Part model, mm, in its own coordinate system. A direction names the side the tool comes from. Give positions to 0.01 mm unless a question says otherwise; leave off trailing zeros. Order: outer loops, then holes, each group sorted by start corner. A loop starts at its lowest first (then second) coordinate and runs counter-clockwise, first axis right, second up. Notation, with made-up numbers: (-6, 71) - (27, 71) arc R15 ccw to (27, 97) - close; hole circle Ø3 at (-27.75, 81.5). An arc over 180 degrees is marked (long way). Use one line per item in the form item = value. Start each with the question number.
1. Pin check, flat tips, straight feed: P1, Ø1.5, axis at x = 13.5, z = 2, coming from the +Y side; P2, Ø1, axis at x = -8.5, z = 2.5, coming from the +Y side; P3, Ø1.5, axis at x = 33.5, z = 3, coming from the +Y side. Stop position of each tip, or through.
2. Tool access for faces 3 (the face through (59, 39, 1)), 4 (the face through (14, 43, 4)): list every direction of +Z, -Z, +X, -X, +Y, -Y with a clear straight run to the whole face (end or side of a thin tool).
3. Pull direction X, two halves, no side cores. Call faces 1 (the face through (-17.24, 37.82, 2.48)), 2 (the face through (14, 43, 0)): +X half, -X half, draft (parallel to the pull), parting line (faces both ways), or undercut.
4. Band-saw the part on B-B, the plane y = 25.5. List the corners of the cut face in (x, z), plus the area to 3 significant figures.
5. Drill centre lines: line 1 (X direction, y = 31.5, z = 1.15); line 2 (Y direction, x = 48, z = 3.4); line 3 (X direction, y = 30, z = 2.5). Where is each one in solid material? Low to high.
6. Band-saw the part on A-A, the plane z = 2. List the corners of the cut face in (x, y), plus the area to 3 significant figures.
from build123d import *

# Parameters (mm, degrees)
F1_DEPTH = 4
F2_DEPTH = 1


with BuildPart() as f1:
    # F0 (on Top) → F1 (new body)
    with BuildSketch(Plane.XY):
        with BuildLine():
            ThreePointArc((33.96875, 44.7240123715), (35.4798914594, 41.6976549267), (36, 38.3552194374))
            ThreePointArc((36, 38.3552194374), (35.4798914594, 35.0127839481), (33.96875, 31.9864265033))
            ThreePointArc((33.96875, 31.9864265033), (34.890304672, 30.0329837344), (36.04875, 28.2100174464))
            ThreePointArc((36.04875, 28.2100174464), (38.9773253879, 32.9114730252), (40, 38.3552194374))
            ThreePointArc((40, 38.3552194374), (38.9773253879, 43.7989658495), (36.04875, 48.5004214283))
            ThreePointArc((36.04875, 48.5004214283), (34.890304672, 46.6774551404), (33.96875, 44.7240123715))
        make_face()
        with BuildLine():
            ThreePointArc((31.92, 46.9058685355), (33.0189287452, 45.8849459782), (33.96875, 44.7240123715))
            ThreePointArc((33.96875, 44.7240123715), (34.890304672, 46.6774551404), (36.04875, 48.5004214283))
            ThreePointArc((36.04875, 48.5004214283), (35.0671824784, 49.4751041915), (34, 50.3552194374))
            ThreePointArc((34, 50.3552194374), (32.8729423014, 48.6830408238), (31.92, 46.9058685355))
        make_face()
        with BuildLine():
            ThreePointArc((36.04875, 28.2100174464), (34.890304672, 30.0329837344), (33.96875, 31.9864265033))
            ThreePointArc((33.96875, 31.9864265033), (33.0189287452, 30.8254928966), (31.92, 29.8045703392))
            ThreePointArc((31.92, 29.8045703392), (32.8729423014, 28.027398051), (34, 26.3552194374))
            ThreePointArc((34, 26.3552194374), (35.0671824784, 27.2353346832), (36.04875, 28.2100174464))
        make_face()
        with BuildLine():
            ThreePointArc((18.08, 46.9058685355), (25, 49.3552194374), (31.92, 46.9058685355))
            ThreePointArc((31.92, 46.9058685355), (32.8729423014, 48.6830408238), (34, 50.3552194374))
            ThreePointArc((34, 50.3552194374), (25, 53.3552194374), (16, 50.3552194374))
            ThreePointArc((16, 50.3552194374), (17.1270576986, 48.6830408238), (18.08, 46.9058685355))
        make_face()
        with BuildLine():
            ThreePointArc((39.8607042186, 52.31076246), (37.804989803, 50.5553926449), (36.04875, 48.5004214283))
            ThreePointArc((36.04875, 48.5004214283), (38.9773253879, 43.7989658495), (40, 38.3552194374))
            ThreePointArc((40, 38.3552194374), (38.9773253879, 32.9114730252), (36.04875, 28.2100174464))
            ThreePointArc((36.04875, 28.2100174464), (37.8049899077, 26.1550461251), (39.8607044582, 24.3996762406))
            ThreePointArc((39.8607044582, 24.3996762406), (38.8098535793, 31.0344868958), (45.4446642345, 32.0853377748))
            ThreePointArc((45.4446642345, 32.0853377748), (42.25, 38.3552195837), (45.4446644712, 44.625101272))
            ThreePointArc((45.4446644712, 44.625101272), (38.8098537523, 45.6759517408), (39.8607042186, 52.31076246))
        make_face()
        with BuildLine():
            ThreePointArc((34, 50.3552194374), (35.0671824784, 49.4751041915), (36.04875, 48.5004214283))
            ThreePointArc((36.04875, 48.5004214283), (37.804989803, 50.5553926449), (39.8607042186, 52.31076246))
            ThreePointArc((39.8607042186, 52.31076246), (57.8313360218, 53.7250820299), (67.25, 38.3552194374))
            ThreePointArc((67.25, 38.3552194374), (57.8313361537, 22.985356912), (39.8607044582, 24.3996762406))
            ThreePointArc((39.8607044582, 24.3996762406), (37.8049899077, 26.1550461251), (36.04875, 28.2100174464))
            ThreePointArc((36.04875, 28.2100174464), (35.0671824784, 27.2353346832), (34, 26.3552194374))
            ThreePointArc((34, 26.3552194374), (37.3874296651, 22.8335227019), (41.5277360562, 20.2383559211))
            ThreePointArc((41.5277360562, 20.2383559211), (43.9514682435, 19.5144497823), (46.3436548255, 18.6922812041))
            ThreePointArc((46.3436548255, 18.6922812041), (62.7842304522, 22.9746000823), (70, 38.3552194374))
            ThreePointArc((70, 38.3552194374), (62.7842304522, 53.7358387924), (46.3436548255, 58.0181576706))
            ThreePointArc((46.3436548255, 58.0181576706), (43.9514682435, 57.1959890924), (41.5277360562, 56.4720829536))
            ThreePointArc((41.5277360562, 56.4720829536), (37.3874296651, 53.8769161728), (34, 50.3552194374))
        make_face()
        with BuildLine():
            ThreePointArc((34, 26.3552194374), (32.8729423014, 28.027398051), (31.92, 29.8045703392))
            ThreePointArc((31.92, 29.8045703392), (25, 27.3552194374), (18.08, 29.8045703392))
            ThreePointArc((18.08, 29.8045703392), (17.1270576986, 28.027398051), (16, 26.3552194374))
            ThreePointArc((16, 26.3552194374), (25, 23.3552194374), (34, 26.3552194374))
        make_face()
        with BuildLine():
            ThreePointArc((16.03125, 44.7240123715), (16.9810712548, 45.8849459782), (18.08, 46.9058685355))
            ThreePointArc((18.08, 46.9058685355), (17.1270576986, 48.6830408238), (16, 50.3552194374))
            ThreePointArc((16, 50.3552194374), (14.9328175216, 49.4751041915), (13.95125, 48.5004214283))
            ThreePointArc((13.95125, 48.5004214283), (15.109695328, 46.6774551404), (16.03125, 44.7240123715))
        make_face()
        with BuildLine():
            ThreePointArc((16, 50.3552194374), (25, 53.3552194374), (34, 50.3552194374))
            ThreePointArc((34, 50.3552194374), (37.3874296651, 53.8769161728), (41.5277360562, 56.4720829536))
            ThreePointArc((41.5277360562, 56.4720829536), (25, 54.228538177), (8.4722639438, 56.4720829536))
            ThreePointArc((8.4722639438, 56.4720829536), (12.6125703349, 53.8769161728), (16, 50.3552194374))
        make_face()
        with BuildLine():
            ThreePointArc((16, 26.3552194374), (17.1270576986, 28.027398051), (18.08, 29.8045703392))
            ThreePointArc((18.08, 29.8045703392), (16.9810712548, 30.8254928966), (16.03125, 31.9864265033))
            ThreePointArc((16.03125, 31.9864265033), (15.109695328, 30.0329837344), (13.95125, 28.2100174464))
            ThreePointArc((13.95125, 28.2100174464), (14.9328175216, 27.2353346832), (16, 26.3552194374))
        make_face()
        with BuildLine():
            ThreePointArc((41.5277360562, 20.2383559211), (37.3874296651, 22.8335227019), (34, 26.3552194374))
            ThreePointArc((34, 26.3552194374), (25, 23.3552194374), (16, 26.3552194374))
            ThreePointArc((16, 26.3552194374), (12.6125703349, 22.8335227019), (8.4722639438, 20.2383559211))
            ThreePointArc((8.4722639438, 20.2383559211), (25, 22.4819006978), (41.5277360562, 20.2383559211))
        make_face()
        with BuildLine():
            ThreePointArc((16.03125, 31.9864265033), (14, 38.3552194374), (16.03125, 44.7240123715))
            ThreePointArc((16.03125, 44.7240123715), (15.109695328, 46.6774551404), (13.95125, 48.5004214283))
            ThreePointArc((13.95125, 48.5004214283), (10, 38.3552194374), (13.95125, 28.2100174464))
            ThreePointArc((13.95125, 28.2100174464), (15.109695328, 30.0329837344), (16.03125, 31.9864265033))
        make_face()
        with BuildLine():
            ThreePointArc((13.95125, 48.5004214283), (14.9328175216, 49.4751041915), (16, 50.3552194374))
            ThreePointArc((16, 50.3552194374), (12.6125703349, 53.8769161728), (8.4722639438, 56.4720829536))
            ThreePointArc((8.4722639438, 56.4720829536), (6.0485317565, 57.1959890924), (3.6563451745, 58.0181576706))
            ThreePointArc((3.6563451745, 58.0181576706), (-20, 38.3552194374), (3.6563451745, 18.6922812041))
            ThreePointArc((3.6563451745, 18.6922812041), (6.0485317565, 19.5144497823), (8.4722639438, 20.2383559211))
            ThreePointArc((8.4722639438, 20.2383559211), (12.6125703349, 22.8335227019), (16, 26.3552194374))
            ThreePointArc((16, 26.3552194374), (14.9328175216, 27.2353346832), (13.95125, 28.2100174464))
            ThreePointArc((13.95125, 28.2100174464), (12.1950101323, 26.1550461651), (10.1392956333, 24.3996763071))
            ThreePointArc((10.1392956333, 24.3996763071), (-17.25, 38.3552194393), (10.1392956365, 52.3107625653))
            ThreePointArc((10.1392956365, 52.3107625653), (12.1950101337, 50.5553927082), (13.95125, 48.5004214283))
        make_face()
        with BuildLine():
            ThreePointArc((50, 46.1052194374), (47.6051183973, 45.7259074724), (45.4446644712, 44.625101272))
            ThreePointArc((45.4446644712, 44.625101272), (42.25, 38.3552195837), (45.4446642345, 32.0853377748))
            ThreePointArc((45.4446642345, 32.0853377748), (53.5184263398, 31.449918858), (57.75, 38.3552194374))
            ThreePointArc((57.75, 38.3552194374), (55.4800775542, 43.8352969916), (50, 46.1052194374))
        make_face()
        with BuildLine():
            ThreePointArc((13.95125, 28.2100174464), (10, 38.3552194374), (13.95125, 48.5004214283))
            ThreePointArc((13.95125, 48.5004214283), (12.1950101337, 50.5553927082), (10.1392956365, 52.3107625653))
            ThreePointArc((10.1392956365, 52.3107625653), (11.5795966532, 50.6243867219), (12.0973156537, 48.4679318671))
            ThreePointArc((12.0973156537, 48.4679318671), (9.503770504, 44.2356508652), (4.5553356627, 44.6251011747))
            ThreePointArc((4.5553356627, 44.6251011747), (6.9053005505, 41.8736458338), (7.75, 38.3552194374))
            ThreePointArc((7.75, 38.3552194374), (6.9053005928, 34.8367931239), (4.5553358133, 32.0853378094))
            ThreePointArc((4.5553358133, 32.0853378094), (9.5037705869, 32.4747879673), (12.0973156537, 28.2425070077))
            ThreePointArc((12.0973156537, 28.2425070077), (11.5795966523, 26.0860521511), (10.1392956333, 24.3996763071))
            ThreePointArc((10.1392956333, 24.3996763071), (12.1950101323, 26.1550461651), (13.95125, 28.2100174464))
        make_face()
        with BuildLine():
            ThreePointArc((7.75, 38.3552194374), (6.9053005505, 41.8736458338), (4.5553356627, 44.6251011747))
            ThreePointArc((4.5553356627, 44.6251011747), (2.3948816814, 45.7259074468), (0, 46.1052194374))
            ThreePointArc((0, 46.1052194374), (-7.3706879807, 35.9603376675), (4.5553358133, 32.0853378094))
            ThreePointArc((4.5553358133, 32.0853378094), (6.9053005928, 34.8367931239), (7.75, 38.3552194374))
        make_face()
    extrude(amount=F1_DEPTH)

    # F0 (on Top) → F2 (join)
    with BuildSketch(Plane.XY):
        with BuildLine():
            ThreePointArc((67.25, 38.3552194374), (57.8313360218, 53.7250820299), (39.8607042186, 52.31076246))
            ThreePointArc((39.8607042186, 52.31076246), (44.8091391214, 52.7002129073), (47.4026843463, 48.4679318671))
            ThreePointArc((47.4026843463, 48.4679318671), (46.8849653857, 46.3114770905), (45.4446644712, 44.625101272))
            ThreePointArc((45.4446644712, 44.625101272), (47.6051183973, 45.7259074724), (50, 46.1052194374))
            ThreePointArc((50, 46.1052194374), (55.4800775542, 43.8352969916), (57.75, 38.3552194374))
            ThreePointArc((57.75, 38.3552194374), (53.5184263398, 31.449918858), (45.4446642345, 32.0853377748))
            ThreePointArc((45.4446642345, 32.0853377748), (46.8849653193, 30.3989619146), (47.4026843463, 28.2425070077))
            ThreePointArc((47.4026843463, 28.2425070077), (44.8091392533, 24.0102260347), (39.8607044582, 24.3996762406))
            ThreePointArc((39.8607044582, 24.3996762406), (57.8313361537, 22.985356912), (67.25, 38.3552194374))
        make_face()
        with BuildLine():
            ThreePointArc((47.4026843463, 48.4679318671), (44.8091391214, 52.7002129073), (39.8607042186, 52.31076246))
            ThreePointArc((39.8607042186, 52.31076246), (38.8098537523, 45.6759517408), (45.4446644712, 44.625101272))
            ThreePointArc((45.4446644712, 44.625101272), (46.8849653857, 46.3114770905), (47.4026843463, 48.4679318671))
        make_face()
        with BuildLine():
            ThreePointArc((45.4446642345, 32.0853377748), (38.8098535793, 31.0344868958), (39.8607044582, 24.3996762406))
            ThreePointArc((39.8607044582, 24.3996762406), (44.8091392533, 24.0102260347), (47.4026843463, 28.2425070077))
            ThreePointArc((47.4026843463, 28.2425070077), (46.8849653193, 30.3989619146), (45.4446642345, 32.0853377748))
        make_face()
        with BuildLine():
            ThreePointArc((4.5553356627, 44.6251011747), (3.5044849583, 51.2599118539), (10.1392956365, 52.3107625653))
            ThreePointArc((10.1392956365, 52.3107625653), (-17.25, 38.3552194393), (10.1392956333, 24.3996763071))
            ThreePointArc((10.1392956333, 24.3996763071), (3.5044849025, 25.4505270977), (4.5553358133, 32.0853378094))
            ThreePointArc((4.5553358133, 32.0853378094), (-7.3706879807, 35.9603376675), (0, 46.1052194374))
            ThreePointArc((0, 46.1052194374), (2.3948816814, 45.7259074468), (4.5553356627, 44.6251011747))
        make_face()
        with BuildLine():
            ThreePointArc((12.0973156537, 48.4679318671), (11.5795966532, 50.6243867219), (10.1392956365, 52.3107625653))
            ThreePointArc((10.1392956365, 52.3107625653), (3.5044849583, 51.2599118539), (4.5553356627, 44.6251011747))
            ThreePointArc((4.5553356627, 44.6251011747), (9.503770504, 44.2356508652), (12.0973156537, 48.4679318671))
        make_face()
        with BuildLine():
            ThreePointArc((4.5553358133, 32.0853378094), (3.5044849025, 25.4505270977), (10.1392956333, 24.3996763071))
            ThreePointArc((10.1392956333, 24.3996763071), (11.5795966523, 26.0860521511), (12.0973156537, 28.2425070077))
            ThreePointArc((12.0973156537, 28.2425070077), (9.5037705869, 32.4747879673), (4.5553358133, 32.0853378094))
        make_face()
    extrude(amount=F2_DEPTH)


solid = f1.part
From the geometry:
q1.P1 = 55.45
q1.P2 = 56.69
q1.P3 = 54.92
q2.face_3 = +Z
q2.face_4 = +Z, +X, -X, +Y, -Y
q3.face_1 = undercut
q3.face_2 = draft
q4.outline = (-15.32, 0) - (65.32, 0) - (65.32, 4) - (61.5, 4) - (61.5, 1) - (38.77, 1) - (38.77, 4) - (11.23, 4) - (11.23, 1) - (-11.5, 1) - (-11.5, 4) - (-15.32, 4) - close
q4.area = 186 mm²
q5.line_1 = -18.79 to -15.83, -3.62 to 3.62, 10.8 to 16.4, 33.6 to 39.2, 46.38 to 53.62, 65.83 to 68.79
q5.line_2 = 18.46 to 21.22, 30.87 to 45.84, 55.49 to 58.25
q5.line_3 = -18.17 to -15.09, 11.76 to 17.85, 32.15 to 38.24, 65.09 to 68.17
q6.outline = (3.66, 18.69) arc R62 cw to (46.34, 18.69) arc R20 ccw (long way) to (46.34, 58.02) arc R62 cw to (3.66, 58.02) arc R20 ccw (long way) to start; hole (4.56, 32.09) arc R7.75 cw (long way) to (4.56, 44.63) arc R4.75 ccw to (10.14, 52.31) arc R17.25 ccw (long way) to (10.14, 24.4) arc R4.75 ccw to start; hole circle Ø22 at (25, 38.36); hole (39.86, 24.4) arc R17.25 ccw (long way) to (39.86, 52.31) arc R4.75 ccw to (45.44, 44.63) arc R7.75 cw (long way) to (45.44, 32.09) arc R4.75 ccw to start
q6.area = 1,440 mm²
